For this review, take the finished solid that the model builds, in its own axes (mm). A direction names the side the tool comes from. Give positions to 0.01 mm unless a question says otherwise; leave off trailing zeros. Write each loop counter-clockwise with the first axis right and the second up, starting at its lowest first coordinate (ties: lowest second). Pieces come first, ordered by that corner, then holes. Notation, with made-up numbers: M 0.5,27 L 11.5,27 A22 ccw 11.5,54 Z; hole C 7,-33 d9. An arc over 180 degrees is marked long. One line per item, written item: value. Start each with the question number.
Item 1: Tool access review of faces 5 (the face through (10, 62, -60.794)), 6 (the face through (10, 36, 99.206)), 7 (the face through (10, 173, 39.206)), 8 (the face through (10, 161, 0.206)): name each direction out of +Z, -Z, +X, -X, +Y, -Y from which nothing blocks a thin tool from reaching the whole face with its end or side.
Item 2: Consider section A-A, the plane z = 65. Write out the cut boundary in (x, y).
Item 3: Consider section D-D, the plane y = 28.5. Write out the cut boundary in (x, z), and give its area (3 significant figures).
Item 4: Mouldability with a two-part tool opening along Z and no side actions: class faces 1 (the face through (10, 161, 19.206)), 2 (the face through (10, 20, 49)), 3 (the face through (9.86, 62.14, 109.066)), 4 (the face through (9.86, 160.74, -40.58)) as released by +Z, released by -Z, zero draft, split by the parting line, or undercut.
Item 5: To check wall thickness, follow probe 1 along Y at (x, z) = (14.5, 97); probe 2 along Y at (x, z) = (7.25, 6); probe 3 along Y at (x, z) = (11.5, 53). State the ranges of each line that lie inside material, in increasing order.
Item 6: Consider section C-C, the plane y = 192. Write out the cut boundary in (x, z).
Item 7: Consider section B-B, the plane x = 6.5. Write out the cut boundary in (y, z).
Item 8: Clearance check with flat-ended pins moving along their axes: pin 1 Ø5.5 at (x, z) = (15, 10) entering from -Y; pin 2 Ø6 at (x, y) = (7, 170) entering from +Z; pin 3 Ø6 at (x, y) = (14.5, 168) entering from -Z. State where each tip first meets the part, or that it passes through.
```python
from build123d import *

# Parameters (mm, degrees)
F0_W     = 180
F0_H     = 19
F1_DEPTH = 20


with BuildPart() as f1:
    # F0 (on Right) → F1 (new body)
    with BuildSketch(Plane.YZ):
        Polygon((52, 99.206252), (52, -60.793748), (72, -60.793748), (252, -19.793748), (272, 0.206252), (272, 19.206252), (252, 39.206252), (92, 39.206252), (72, 59.206252), (72, 99.206252), (52, 119.206252), (20, 119.206252), (0, 99.206252), (0, 19.206252), (20, -0.793748), (20, 99.206252), align=None)
        with Locations((162, 9.706252)):
            Rectangle(F0_W, F0_H, mode=Mode.SUBTRACT)
    extrude(amount=F1_DEPTH)


solid = f1.part
```
Model answer:
1. face 5: -Z, +X, -X, +Y, -Y
1. face 6: -Z, +X, -X
1. face 7: +Z, +X, -X, +Y
1. face 8: +X, -X
2. outline: M 0,0 L 20,0 L 20,20 L 0,20 Z; M 0,52 L 20,52 L 20,72 L 0,72 Z
3. outline: M 0,99.21 L 20,99.21 L 20,119.21 L 0,119.21 Z
3. area: 400 mm2
4. face 1: undercut
4. face 2: zero draft
4. face 3: released by +Z
4. face 4: released by -Z
5. probe 1: y = 0 to 20, 52 to 72
5. probe 2: y = 13.21 to 20, 52 to 72, 252 to 272
5. probe 3: y = 0 to 20, 52 to 78.21
6. outline: M 0,-33.46 L 20,-33.46 L 20,0.21 L 0,0.21 Z; M 0,19.21 L 20,19.21 L 20,39.21 L 0,39.21 Z
7. outline: M 0,19.21 L 20,-0.79 L 20,99.21 L 52,99.21 L 52,-60.79 L 72,-60.79 L 252,-19.79 L 272,0.21 L 272,19.21 L 252,39.21 L 92,39.21 L 72,59.21 L 72,99.21 L 52,119.21 L 20,119.21 L 0,99.21 Z; hole M 72,0.21 L 252,0.21 L 252,19.21 L 72,19.21 Z
8. pin 1: stops at y = 6.46
8. pin 2: stops at z = 39.21
8. pin 3: stops at z = -39.61
